Check sheet for the modelled part. Datum: model origin and axes. Units: mm. A direction names the side the tool comes from. Coordinates: 2 decimals unless noted, no trailing zeros. Order: outer loops, then holes, each group sorted by start corner. A loop starts at its lowest first (then second) coordinate and runs counter-clockwise, first axis right, second up. Notation, with made-up numbers: (81, -17) -> (129, -17) arc R23 cw to (129, 22) -> close; hole circle Ø11 at (-29.5, -9.5). An arc over 180 degrees is marked (long way). Put each result on its own line as item: value. Start each with the question number.
```python
from build123d import *

# Parameters (mm, degrees)
SKETCH1_W           = 69.85
SKETCH1_H           = 69.85
BOSS_EXTRUDE1_DEPTH = 76.2
SKETCH2_R           = 13.716
CUT_EXTRUDE1_DEPTH  = 76.2
SKETCH4_R           = 21.209
CUT_EXTRUDE2_DEPTH  = 17.018
SKETCH5_R           = 21.209
CUT_EXTRUDE3_DEPTH  = 7.62


with BuildPart() as part:
    # Sketch1 → Boss-Extrude1 (new body)
    with BuildSketch(Plane(origin=(0, 0, 0), x_dir=(1, 0, 0), z_dir=(0, 1, 0))):
        with Locations((34.925, 34.925)):
            Rectangle(SKETCH1_W, SKETCH1_H)
    extrude(amount=BOSS_EXTRUDE1_DEPTH)

    # Sketch2 → Cut-Extrude1 (cut)
    with BuildSketch(Plane(origin=(0, 76.2, 0), x_dir=(1, 0, 0), z_dir=(0, 1, 0))):
        with Locations((34.925, 34.925)):
            Circle(SKETCH2_R)
    extrude(amount=-CUT_EXTRUDE1_DEPTH, mode=Mode.SUBTRACT)

    # Sketch4 → Cut-Extrude2 (cut)
    with BuildSketch(Plane(origin=(0, 76.2, 0), x_dir=(1, 0, 0), z_dir=(0, 1, 0))):
        with Locations((34.925, 34.925)):
            Circle(SKETCH4_R)
    extrude(amount=-CUT_EXTRUDE2_DEPTH, mode=Mode.SUBTRACT)

    # Sketch5 → Cut-Extrude3 (cut)
    with BuildSketch(Plane.XZ):
        with Locations((34.925, -34.925)):
            Circle(SKETCH5_R)
    extrude(amount=-CUT_EXTRUDE3_DEPTH, mode=Mode.SUBTRACT)


solid = part.part
```
1) Sectioned sample at A-A (x = 32). Record the boundary of the cut face in (y, z).
2) Sectioned sample at C-C (y = 38.5). Record the boundary of the cut face in (x, z) (3 decimals).
3) Sectioned sample at B-B (z = -37). Record the boundary of the cut face in (x, y), plus the area to 3 significant figures.
4) Mould release check, pull along X, two halves, no side actions. Record for faces 1 (the flat face through (0, 38, -34)), 2 (the flat face through (34, 38, 0)), 3 (the cylindrical face through (46.327, 67.81, -52.809)): +X half, -X half, draft (parallel to the pull), parting line (faces both ways), or undercut.
5) Scan lines: line 1 along X through (y, z) = (40, -37); line 2 along X through (y, z) = (12, -45.5); line 3 along Z through (x, y) = (18, 62). Record each from-to range of solid material in increasing order. Write a range as [from, to].
6) Gauge pin test, flat ends, axial feed: pin 1 (8 mm diameter, centred on x = 34, z = -50.5, fed in from +Y); pin 2 (5 mm diameter, centred on x = 31.5, z = -22.5, fed in from -Y); pin 3 (12.5 mm diameter, centred on x = 41.5, z = -33.5, fed in from +Y). Record the tip position at first contact, or that the pin passes through.
7) Sectioned sample at D-D (x = 53.5). Record the boundary of the cut face in (y, z), plus the area to 3 significant figures.
8) Access from +Z, -Z, +X, -X, +Y, -Y to the whole of each face (thin tool, end or side, straight path). Record for faces 4 (the flat face through (49, 59.182, -35)), 5 (the flat face through (50, 0, -51)), 6 (the flat face through (35, 7.62, -49)).
Entries:
1. outline: (0, -69.85) -> (76.2, -69.85) -> (76.2, -55.93) -> (59.18, -55.93) -> (59.18, -48.33) -> (7.62, -48.33) -> (7.62, -55.93) -> (0, -55.93) -> close; (0, -13.92) -> (7.62, -13.92) -> (7.62, -21.52) -> (59.18, -21.52) -> (59.18, -13.92) -> (76.2, -13.92) -> (76.2, 0) -> (0, 0) -> close
2. outline: (0, -69.85) -> (69.85, -69.85) -> (69.85, 0) -> (0, 0) -> close; hole circle Ø27.432 at (34.925, -34.925)
3. outline: (0, 0) -> (13.82, 0) -> (13.82, 7.62) -> (21.37, 7.62) -> (21.37, 59.18) -> (13.82, 59.18) -> (13.82, 76.2) -> (0, 76.2) -> close; (48.48, 7.62) -> (56.03, 7.62) -> (56.03, 0) -> (69.85, 0) -> (69.85, 76.2) -> (56.03, 76.2) -> (56.03, 59.18) -> (48.48, 59.18) -> close
3. area: 2,880 mm2
4. face 1: -X half
4. face 2: draft
4. face 3: undercut
5. line 1: x = [0, 21.37], [48.48, 69.85]
5. line 2: x = [0, 26.19], [43.66, 69.85]
5. line 3: z = [-69.85, -47.71], [-22.14, 0]
6. pin 1: stops at y = 59.18
6. pin 2: stops at y = 7.62
6. pin 3: passes through
7. outline: (0, -69.85) -> (76.2, -69.85) -> (76.2, -45.16) -> (59.18, -45.16) -> (59.18, -24.69) -> (76.2, -24.69) -> (76.2, 0) -> (0, 0) -> (0, -24.69) -> (7.62, -24.69) -> (7.62, -45.16) -> (0, -45.16) -> close
7. area: 4,820 mm2
8. face 4: +Y
8. face 5: +Z, -Z, +X, -X, -Y
8. face 6: -Y
